from build123d import *

# Parameters (mm, degrees)
EXTRUDE_1_DEPTH          = 10
SHELL_START              = 1
SHELL_5_DEPTH            = 9
CUT_EXTRUDE_1_DEPTH      = 134.004728562
CUT_EXTRUDE_1_DEPTH_BACK = 134.004728562
SKETCH_2_R               = 1.6
SKETCH_6_W               = 20.772573636
SKETCH_6_H               = 20.357122163
CUT_EXTRUDE_2_DEPTH      = 104.896631765
CUT_EXTRUDE_3_REACH      = 105.897
SKETCH_9_R               = 2


# Read off the part's stored shape, not the designer's step: 薄殼5
with BuildPart() as part:
    # 草圖1 → 填料-伸長1 (new body)
    with BuildSketch(Plane(origin=(0, 0, 0), x_dir=(1, 0, 0), z_dir=(0, 1, 0))):
        with BuildLine():
            Line((-41.238095238, 59.166666667), (-41.238095238, -70.833333333))
            ThreePointArc((-41.238095238, -70.833333333), (-38.016269831, -78.611507926), (-30.238095238, -81.833333333))
            Line((-30.238095238, -81.833333333), (49.761904762, -81.833333333))
            ThreePointArc((49.761904762, -81.833333333), (58.868802246, -79.414212178), (62.761904762, -70.833333333))
            Line((62.761904762, -70.833333333), (62.761904762, 59.166666667))
            ThreePointArc((62.761904762, 59.166666667), (59.768077482, 69.172839387), (49.761904762, 72.166666667))
            Line((49.761904762, 72.166666667), (-30.238095238, 72.166666667))
            ThreePointArc((-30.238095238, 72.166666667), (-38.818974083, 68.273564151), (-41.238095238, 59.166666667))
        make_face()
    extrude(amount=EXTRUDE_1_DEPTH)

    # 薄殼5 outline → 薄殼5 (cut)
    with BuildSketch(Plane(origin=(0, 0, 0), x_dir=(1, 0, 0), z_dir=(0, 1, 0)).offset(SHELL_START)):
        with BuildLine():
            ThreePointArc((-30.246641499, 71.166666667), (-38.08182369, 67.59648754), (-40.238095238, 59.260616141))
            Line((-40.238095238, 59.260616141), (-40.238095238, -70.833333333))
            ThreePointArc((-40.238095238, -70.833333333), (-37.30916305, -77.904401145), (-30.238095238, -80.833333333))
            Line((-30.238095238, -80.833333333), (49.855854237, -80.833333333))
            ThreePointArc((49.855854237, -80.833333333), (58.191725636, -78.677061785), (61.761904762, -70.841879594))
            Line((61.761904762, -70.841879594), (61.761904762, 59.271464521))
            ThreePointArc((61.761904762, 59.271464521), (59.060970701, 68.465732606), (49.866702616, 71.166666667))
            Line((49.866702616, 71.166666667), (-30.246641499, 71.166666667))
        make_face()
    extrude(amount=SHELL_5_DEPTH, mode=Mode.SUBTRACT)

    # 草圖2 → 除料-伸長1 (cut, two sides: drawn at the far end of the back side and taken through both)
    with BuildSketch(Plane.ZY.offset(41.238095238).offset(-CUT_EXTRUDE_1_DEPTH_BACK)):
        with Locations((-51.166666667, 5)):
            Circle(SKETCH_2_R)
        with Locations((58.833333333, 5)):
            Circle(SKETCH_2_R)
    extrude(amount=CUT_EXTRUDE_1_DEPTH + CUT_EXTRUDE_1_DEPTH_BACK, mode=Mode.SUBTRACT)

    # 草圖6 → 除料-伸長2 (cut, through all)
    with BuildSketch(Plane(origin=(0, 0, 0), x_dir=(-1, 0, 0), z_dir=(0, -1, 0))):
        with Locations((-10.761904762, -61.833333334)):
            Rectangle(SKETCH_6_W, SKETCH_6_H)
    extrude(amount=-CUT_EXTRUDE_2_DEPTH, mode=Mode.SUBTRACT)

    # 草圖9 → 除料-伸長3 (cut, up to next)
    with BuildSketch(Plane.XZ, mode=Mode.PRIVATE) as cut_extrude_3_sk1:
        with Locations(Location((-14.488095238, -43.164036493, 0), (0, 0, 270))):
            Circle(SKETCH_9_R)
    cut_extrude_3_tool1 = extrude(cut_extrude_3_sk1.sketch, amount=-CUT_EXTRUDE_3_REACH, mode=Mode.PRIVATE) & part.part
    # 草圖9 → 除料-伸長3 (cut, up to next)
    with BuildSketch(Plane.XZ, mode=Mode.PRIVATE) as cut_extrude_3_sk2:
        with Locations(Location((34.011904762, -43.164036493, 0), (0, 0, 90))):
            Circle(SKETCH_9_R)
    cut_extrude_3_tool2 = extrude(cut_extrude_3_sk2.sketch, amount=-CUT_EXTRUDE_3_REACH, mode=Mode.PRIVATE) & part.part
    # 草圖9 → 除料-伸長3 (cut, up to next)
    with BuildSketch(Plane.XZ, mode=Mode.PRIVATE) as cut_extrude_3_sk3:
        with Locations(Location((9.761904762, -43.164036493, 0), (0, 0, 270))):
            Circle(SKETCH_9_R)
    cut_extrude_3_tool3 = extrude(cut_extrude_3_sk3.sketch, amount=-CUT_EXTRUDE_3_REACH, mode=Mode.PRIVATE) & part.part
    add(cut_extrude_3_tool1.solids().sort_by_distance((-14.488095, 0, -43.164036))[0], mode=Mode.SUBTRACT)
    add(cut_extrude_3_tool2.solids().sort_by_distance((34.011905, 0, -43.164036))[0], mode=Mode.SUBTRACT)
    add(cut_extrude_3_tool3.solids().sort_by_distance((9.761905, 0, -43.164036))[0], mode=Mode.SUBTRACT)


solid = part.part
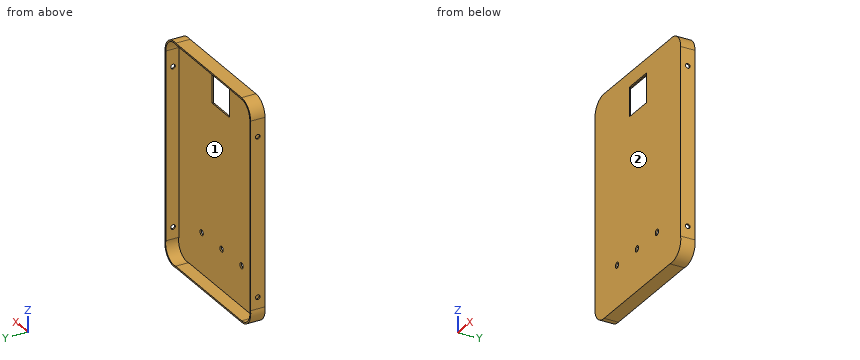
Can you work these out from the model? Positions are in its coordinate system, mm. Face numbers are marked on the shaded views. Give positions to 0.01 mm unless a question says otherwise; leave off trailing zeros. Write each loop counter-clockwise with the first axis right and the second up, starting at its lowest first coordinate (ties: lowest second). Pieces come first, ordered by that corner, then holes. Notation, with made-up numbers: M 63,29.5 L 115,29.5 A20 ccw 115,37.5 Z; hole C -19.5,39.5 d10. An arc over 180 degrees is marked long. Answer in a Markdown table with one row per item. Add a question column.
Item 1: For pin 1 Ø5 at (x, y) = (21, 4) entering from +Z; pin 2 Ø3.5 at (y, z) = (5, 58.83) entering from +X; pin 3 Ø6.5 at (x, z) = (9.76, -43.16) entering from +Y; pin 4 Ø3 at (y, z) = (5, -51.17) entering from -X, each with a flat end and sliding along its axis, tell me the tip position at first contact or that it passes through.
Item 2: Imagine slicing it at C-C, the plane x = 24.5. Write out the boundary of the cut face in (y, z).
Item 3: Imagine slicing it at B-B, the plane z = 21. Write out the boundary of the cut face in (x, y), plus the area to 3 significant figures.
Item 4: Please list where these lines run through material, in increasing order: L1, parallel to Z at x = -23.5, y = 3; L2, parallel to X at y = 4, z = -19; L3, parallel to X at y = 0.5, z = 70.5.
Item 5: Imagine slicing it at A-A, the plane y = 5. State how many separate pieces and enclosed holes the cut face has, plus the area to 3 significant figures.
Item 6: We'd pull the mould along Z, two halves only. Please class the marked faces 1 and 2: released by +Z, released by -Z, zero draft, split by the parting line, or undercut.
Evaluation:
| question | item | result |
|---|---|---|
| 1 | pin 1 | stops at z = 81.83 |
| 1 | pin 2 | stops at x = 62.76 |
| 1 | pin 3 | stops at y = 1 |
| 1 | pin 4 | passes through |
| 2 | outline | M 0,-72.17 L 10,-72.17 L 10,-71.17 L 1,-71.17 L 1,80.83 L 10,80.83 L 10,81.83 L 0,81.83 Z |
| 3 | outline | M -41.24,0 L 62.76,0 L 62.76,10 L 61.76,10 L 61.76,1 L -40.24,1 L -40.24,10 L -41.24,10 Z |
| 3 | area | 122 mm² |
| 4 | L1 | z = -72.17 to -71.17, 80.83 to 81.83 |
| 4 | L2 | x = -41.24 to -40.24, 61.76 to 62.76 |
| 4 | L3 | x = -41.24 to 0.38, 21.15 to 62.76 |
| 5 | separate pieces | 4 |
| 5 | enclosed holes | 0 |
| 5 | area | 482 mm² |
| 6 | face 1 | undercut |
| 6 | face 2 | zero draft |
